Verification items for the finished model (mm, model axes). Face numbers are marked on the shaded views. A direction names the side the tool comes from. Coordinates: 2 decimals unless noted, no trailing zeros. Loops run counter-clockwise (first coordinate to the right, second up) from the corner with the lowest first, then second, coordinate; pieces in that order, holes last. Notation, with made-up numbers: (88, 59.5) - (104, 59.5) arc R17 cw to (104, 63.5) - close; hole circle Ø3 at (-27.75, 47.5). An arc over 180 degrees is marked (long way). Answer as CSV lines item,"result". Start each with the question number.
1. Release check for a two-part mould opening along Z. For the marked faces 1, 2 and 3 record: pulls with the +Z half, pulls with the -Z half, needs draft (parallel to the pull), parting line crosses it, or undercut.
2. Gauge pin test, flat ends, axial feed: P1, Ø10, axis at x = -19, z = -4.5, coming from the +Y side; P2, Ø6, axis at x = 38.5, z = -69, coming from the +Y side. Record the tip position at first contact, or that the pin passes through.
3. Cross-section at C-C (z = -86). Enter the section's corners in (x, y).
4. Cross-section at B-B (x = 0). Enter the section's corners in (y, z).
5. Material ranges on line 1 (Z direction, x = -51.5, y = -140.5); line 2 (Y direction, x = 30, z = -62.5); line 3 (X direction, y = -14.5, z = -91.5), recorded low to high. Write a range as [from, to].
6. Cross-section at D-D (x = -63). Enter the section's corners in (y, z).
7. Set-up check for the marked faces 4 and 5: record each of +Z, -Z, +X, -X, +Y, -Y from which the full face is reachable in a straight line by a thin tool's end or side.
8. Cross-section at A-A (y = -104.5). Enter the section's corners in (x, z), plus the area to 3 significant figures.
Autodesk Inventor part; units mm, degrees
ref_plane "Work Plane1" through (0, 0, -40) normal (0, 0, -1) x (1, 0, 0)
ref_plane "YZ Plane" through (0, 0, 0) normal (1, 0, 0) x (0, 1, 0)
ref_plane "XZ Plane" through (0, 0, 0) normal (0, 1, 0) x (-1, 0, 0)
sketch "Sketch1" plane through (0, 0, 0) normal (0, 0, 1) x (1, 0, 0)
  arc A0 (-87.5, 0) -> (87.5, 0) centre (0, 0) ccw
  line L0 (-87.5, 0) -> (87.5, 0) construction
  line L1 (-87.5, -200) -> (87.5, -200)
  line L2 (-87.5, -220) -> (87.5, -220)
  line L3 (-87.5, 0) -> (-107.5, 0)
  line L4 (0, 0) -> (-107, 0)
  line L5 (-107, 0) -> (-107, -200)
  line L6 (-107, -200) -> (-87.5, -200)
  line L7 (-107, -200) -> (-107, -220)
  line L8 (-107, -220) -> (-87.5, -220)
  line L9 (0, 0) -> (107, 0)
  line L10 (107, 0) -> (107, -220)
  line L11 (107, -220) -> (87.5, -220)
  line L12 (87.5, -200) -> (107, -200)
  point P0 (87.5, 0)
  dimension "d0" = 175
  dimension "d1" = 200
  dimension "d9" = 107
  dimension "d10" = 107
  dimension "d13" = 90
  dimension "d15" = 200
  dimension "d17" = 200
  dimension "d18" = 214.5
  dimension "d21" = 20
extrude "Extrusion1" add sketch "Sketch1" along normal blind 20 contours A0 L9 L10 L12 L1 L6 L5 L3
extrude "Extrusion2" add sketch "Sketch1" along normal blind 20 and the other way blind 100 contours L6 L1 L12 L10 L11 L2 L8 L7
ref_plane "Work Plane1" through (0, 0, -40) normal (0, 0, -1) x (1, 0, 0)
mirror "Mirror1" about plane through (0, 0, -40) normal (0, 0, -1) of "Extrusion1"
properties part number "Support" material "Stainless Steel"
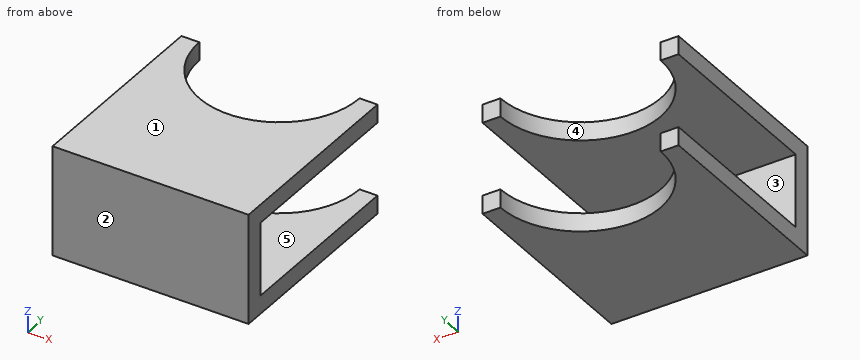
Values follow:
1,face 1,"pulls with the +Z half"
1,face 2,"needs draft"
1,face 3,"undercut"
2,P1,"stops at y = -84.9"
2,P2,"stops at y = -200"
3,outline,"(-107, -220) - (107, -220) - (107, 0) - (87.5, 0) arc R87.5 cw to (-87.5, 0) - (-107, 0) - close"
4,outline,"(-220, -100) - (-87.5, -100) - (-87.5, -80) - (-200, -80) - (-200, 0) - (-87.5, 0) - (-87.5, 20) - (-220, 20) - close"
5,line 1,"z = [-100, -80], [0, 20]"
5,line 2,"y = [-220, -200]"
5,line 3,"x = [-107, -86.29], [86.29, 107]"
6,outline,"(-220, -100) - (-60.72, -100) - (-60.72, -80) - (-200, -80) - (-200, 0) - (-60.72, 0) - (-60.72, 20) - (-220, 20) - close"
7,face 4,"+Z, -Z, +Y"
7,face 5,"+X, -X, +Y"
8,outline,"(-107, -100) - (107, -100) - (107, -80) - (-107, -80) - close; (-107, 0) - (107, 0) - (107, 20) - (-107, 20) - close"
8,area,"8,560 mm²"
